Answer from the drawing. Dimensions are ordinates in mm from the lowest x, y and z of the part. Give positions to 0.01 mm unless a question says otherwise; leave off trailing zeros. Order: outer loops, then holes, each group sorted by start corner. A loop starts at its lowest first (then second) coordinate and runs counter-clockwise, first axis right, second up. Notation, with made-up numbers: (24.25, 59.5) -> (72.25, 59.5) arc R12 cw to (72.25, 71.5) -> close; hole circle Ø4 at (15.25, -17). An arc over 180 degrees is marked (long way). Answer as CSV lines item,"result". Start each with the question number.
1) Flat-ended cylindrical pins translate along their axes: pin 1 Ø3 at (x, z) = (62.5, 101.5) entering from -Y; pin 2 Ø8 at (x, z) = (195.5, 4.5) entering from +Y. Find the tip coordinate at first contact, or state that the pin passes through.
2) Straight lines are drawn through the part: L1, parallel to Z at x = 166, y = 14; L2, parallel to Z at x = 138.5, y = 2.5; L3, parallel to Z at x = 189, y = 4. For each, find the intervals that lie inside material, in ascending order. Write a range as from..to.
3) Find section B-B (x = 104). Determine the outline of the cut face in (y, z).
4) The mould has two halves that part along Z. Classify the marked faces 1 and 2: +Z half, -Z half, draft (parallel to the pull), parting line (faces both ways), or undercut.
5) Find section C-C (y = 3.5). State how many separate pieces and enclosed holes the cut face has, and give its area (3 significant figures).
6) Find section A-A (z = 22). Determine the outline of the cut face in (x, y), and give its area (3 significant figures).
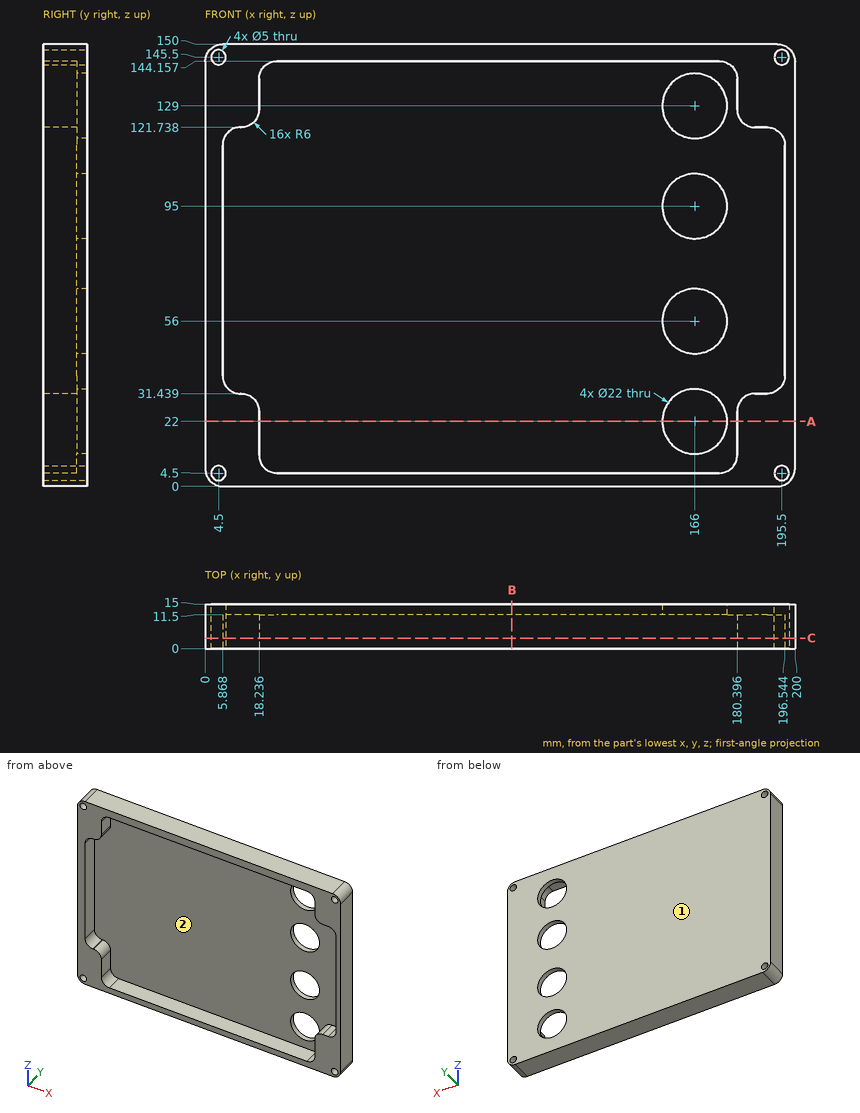
Findings below:
1,pin 1,"y = 11.5"
1,pin 2,"y = 15"
2,L1,"0..11, 33..45, 67..84, 106..118, 140..150"
2,L2,"0..4.5, 144.16..150"
2,L3,"0..31.44, 121.74..150"
3,outline,"(0, 0) -> (15, 0) -> (15, 150) -> (0, 150) -> (0, 144.16) -> (11.5, 144.16) -> (11.5, 4.5) -> (0, 4.5) -> close"
4,face 1,"draft"
4,face 2,"undercut"
5,separate pieces,"1"
5,enclosed holes,"5"
5,area,"4,700 mm²"
6,outline,"(0, 0) -> (18.24, 0) -> (18.24, 11.5) -> (155, 11.5) -> (155, 15) -> (0, 15) -> close; (177, 11.5) -> (180.4, 11.5) -> (180.4, 0) -> (200, 0) -> (200, 15) -> (177, 15) -> close"
6,area,"1,060 mm²"
